Source: CAD feature listing. Evaluate the final solid. Frame: model axes, mm. A direction names the side the tool comes from. Give positions to 0.01 mm unless a question says otherwise; leave off trailing zeros. Order: outer loops, then holes, each group sorted by start corner. A loop starts at its lowest first (then second) coordinate and runs counter-clockwise, first axis right, second up. Notation, with made-up numbers: M -3,-27.75 L 11,-27.75 A24 ccw 11,-13.75 Z; hole C -4,5.25 d6. An arc over 180 degrees is marked long. One line per question, with ' | ' between items. Start each with the question number.
from build123d import *

# Parameters (mm, degrees)
REVOLVE2_ANGLE           = 180
BOSS_EXTRUDE1_DEPTH      = 6.35
BOSS_EXTRUDE1_DEPTH_BACK = 6.35
SKETCH10_W               = 7.62
SKETCH10_H               = 7.62
BOSS_EXTRUDE2_DEPTH      = 6.35


# Read off the part's stored shape, not the designer's step: Revolve2
with BuildPart() as part:
    # Revolve2 outline → Revolve2 (revolve)
    with BuildSketch(Plane.XZ):
        Polygon((3.81, 0), (0, 0), (0, -3.81), (38.1, -41.91), (41.91, -41.91), (41.91, -38.1), align=None)
    revolve(axis=Axis((0, 0, 0), (0, 0, 1)), revolution_arc=REVOLVE2_ANGLE)

    # Sketch6 → Boss-Extrude1 (add, two sides: drawn at the far end of the back side and taken through both)
    with BuildSketch(Plane(origin=(0, 0, 0), x_dir=(0, 0, -1), z_dir=(1, 0, 0)).offset(-BOSS_EXTRUDE1_DEPTH_BACK)):
        Polygon((20.32, 20.32), (20.32, 29.318948776), (20.32, 36.223650293), (30.48, 36.223650293), (30.48, 30.48), align=None)
    extrude(amount=BOSS_EXTRUDE1_DEPTH + BOSS_EXTRUDE1_DEPTH_BACK)

    # Sketch10 → Boss-Extrude2 (add)
    with BuildSketch(Plane(origin=(0, 36.223650293, 0), x_dir=(1, 0, 0), z_dir=(0, 1, 0))):
        with Locations((0, 25.4)):
            Rectangle(SKETCH10_W, SKETCH10_H)
    extrude(amount=BOSS_EXTRUDE2_DEPTH)


solid = part.part
Item 1: Pin query (flat end, axial travel): pin 1 Ø1 at (x, y) = (-13.5, 6) entering from +Z; pin 2 Ø1 at (x, y) = (14.5, 18.5) entering from -Z; pin 3 Ø1.5 at (x, y) = (26, 18.5) entering from +Z; pin 4 Ø12 at (x, z) = (23, -20.5) entering from -Y. Return the tip coordinate at first contact, or that it passes through.
Item 2: Cut plane B-B on z = -26. Return the cut outline in (x, y), and give its area (3 significant figures).
Item 3: Mould query, pull axis Z, two halves, no side actions, for faces 4 (the flat face through (0, 39, -21.59)), 5 (the flat face through (0, 39, -29.21)), 6 (the flat face through (0, 35, -30.48)), 7 (the flat face through (-6.35, 31, -24)). Classes: pulls with the +Z half, pulls with the -Z half, needs draft (parallel to the pull), parting line crosses it, or undercut.
Item 4: Line query: line 1 (X direction, y = 11, z = -29); line 2 (X direction, y = 31, z = -26); line 3 (Z direction, x = 10, y = 4). Output: solid intervals per line, ascending.
Item 5: Reachability of faces 1 (the flat face through (-3.81, 39, -25)), 2 (the flat face through (-10, 0, -13)), 3 (the flat face through (6.35, 31, -24)) from +Z, -Z, +X, -X, +Y, -Y: full face, straight path, thin tool, end or side. Return the list, or none.
Item 6: Cut plane C-C on z = -32.5. Return the cut outline in (x, y).
Item 7: Cut plane A-A on x = 0. Return the cut outline in (y, z), and give its area (3 significant figures).
Results are:
1) pin 1: stops at z = -10.46 | pin 2: stops at z = -27.82 | pin 3: stops at z = -27.35 | pin 4: stops at y = 0
2) outline: M -29.81,0 L -22.19,0 A22.19 cw 22.19,0 L 29.81,0 A29.81 ccw 6.35,29.13 L 6.35,36.22 L 3.81,36.22 L 3.81,42.57 L -3.81,42.57 L -3.81,36.22 L -6.35,36.22 L -6.35,29.13 A29.81 ccw Z | area: 755 mm2
3) face 4: pulls with the +Z half | face 5: undercut | face 6: undercut | face 7: needs draft
4) line 1: x = -30.91 to -22.66, 22.66 to 30.91 | line 2: x = -6.35 to 6.35 | line 3: z = -14.58 to -6.96
5) face 1: +Z, -X, +Y | face 2: +Z, -Z, +X, -X, -Y | face 3: +Z, +X, +Y
6) outline: M -36.31,0 L -28.69,0 A28.69 cw 28.69,0 L 36.31,0 A36.31 ccw Z
7) outline: M 0,-3.81 L 38.1,-41.91 L 41.91,-41.91 L 41.91,-38.1 L 34.29,-30.48 L 36.22,-30.48 L 36.22,-29.21 L 42.57,-29.21 L 42.57,-21.59 L 36.22,-21.59 L 36.22,-20.32 L 24.13,-20.32 L 3.81,0 L 0,0 Z | area: 424 mm2
